CAD build for the part. Positions are in the model's coordinates, mm. A direction names the side the tool comes from. Coordinates: 2 decimals unless noted, no trailing zeros. Loops run counter-clockwise (first coordinate to the right, second up) from the corner with the lowest first, then second, coordinate; pieces in that order, holes last. Notation, with made-up numbers: (-10.75, -26.75) -> (7.25, -26.75) arc R22 ccw to (7.25, 2.25) -> close; hole circle Ø8 at (30, 47). An arc over 180 degrees is marked (long way). Answer as CSV lines item,"result". Start each with the question number.
```python
from build123d import *

# Parameters (mm, degrees)
CONG_1_R = 0.5


with BuildPart() as part:
    # Esquisse1 → Révolution1 (revolve)
    with BuildSketch(Plane.XY, mode=Mode.PRIVATE) as r_volution1_sk:
        with BuildLine():
            Line((-3.5, 13), (4.5, 13))
            Line((4.5, 13), (4.5, 5.5))
            Line((4.5, 5.5), (2.5, 5.5))
            Line((2.5, 5.5), (2.5, 8.5))
            ThreePointArc((2.5, 8.5), (1.767766953, 10.267766953), (0, 11))
            Line((0, 11), (-3.5, 11))
            Line((-3.5, 11), (-3.5, 13))
        make_face()
    revolve(r_volution1_sk.sketch.rotate(Axis((-12.986342457, 0, 0), (1, 0, 0)), 90), axis=Axis((-12.986342457, 0, 0), (1, 0, 0)))  # turned: the seam where the file's is

    # Congé1
    cong_1_edges = [part.edges().sort_by_distance(p)[0] for p in [
        (4.5, 0, -13),
    ]]
    fillet(cong_1_edges, radius=CONG_1_R)


solid = part.part
```
Q1. Which spindle directions (+Z, -Z, +X, -X, +Y, -Y) get a long thin tool onto all of the face, cutting with end or side? Do faces 1 (the flat face through (2.5, 6, 0)), 2 (the cylindrical face through (3.49, 5.37, -1.19)). Say none if no direction does.
Q2. Saw through at C-C (x = -0.5). List the corners of the cut face in (y, z).
Q3. Pin check, flat tips, straight feed: pin 1 Ø4 at (x, y) = (-2, -7) entering from -Z; pin 2 Ø1.5 at (x, z) = (-1, -7.5) entering from +Y. Stop position of each tip, or through.
Q4. Two-plate mould, pull along Z, no slides. Class faces 3 (the cylindrical face through (0.303, 7.91, -10.316)), 4 (the cylindrical face through (-1.77, 10.74, -2.38)), 5 (the flat face through (4.5, 5, 3)): pulls with the +Z half, pulls with the -Z half, needs draft (parallel to the pull), parting line crosses it, or undercut.
Q5. Probe probe 1 along Y at (x, z) = (3.5, 0); probe 2 along Y at (x, z) = (-1, 0); probe 3 along X at (y, z) = (1, -7). List the from-to ranges inside material, lowest first. Write a range as from..to.
Q6. Saw through at A-A (y = 0). List the corners of the cut face in (x, z).
Ans:
1,face 1,"-X"
1,face 2,"+X, -X"
2,outline,"circle Ø26 at (0, 0); hole circle Ø22 at (0, 0)"
3,pin 1,"stops at z = -12"
3,pin 2,"stops at y = 11.11"
4,face 3,"parting line crosses it"
4,face 4,"undercut"
4,face 5,"needs draft"
5,probe 1,"y = -13..-5.5, 5.5..13"
5,probe 2,"y = -13..-11, 11..13"
5,probe 3,"x = 2.5..4.5"
6,outline,"(-3.5, -13) -> (4, -13) arc R0.5 ccw to (4.5, -12.5) -> (4.5, -5.5) -> (2.5, -5.5) -> (2.5, -8.5) arc R2.5 cw to (0, -11) -> (-3.5, -11) -> close; (-3.5, 11) -> (0, 11) arc R2.5 cw to (2.5, 8.5) -> (2.5, 5.5) -> (4.5, 5.5) -> (4.5, 12.5) arc R0.5 ccw to (4, 13) -> (-3.5, 13) -> close"
